Geometry: final body of the model. Coordinates: model frame, mm. Round coordinates to 2 decimals unless told otherwise and drop trailing zeros. Loops run counter-clockwise (first coordinate to the right, second up) from the corner with the lowest first, then second, coordinate; pieces in that order, holes last. Notation, with made-up numbers: (-25, 54.5) - (21, 54.5) arc R9 cw to (21, 70.5) - close; hole circle Ø5 at (32.25, 28). An arc over 180 degrees is marked (long way). Answer as a JSON object with one key per item and string values. Group by question number.
Item 1: Section A-A (z = 70.5). Return the cut outline in (x, y) (1 decimal).
Item 2: First-contact query: pin 1 (3 mm diameter, centred on y = -2, z = 101, fed in from +X); pin 2 (2 mm diameter, centred on x = 3.5, z = -84, fed in from +Y). Flat tips, straight axial feed; report the tip coordinate or a pass-through.
Item 3: Line query: line 1 (X direction, y = 0.25, z = 40.5); line 2 (Y direction, x = 0.75, z = 114); line 3 (X direction, y = -2.75, z = 89). Output: solid intervals per line, ascending.
```python
from build123d import *

# Parameters (mm, degrees)
SKETCH3_R                = 4.7625
BOSS_EXTRUDE2_DEPTH      = 152.4
BOSS_EXTRUDE2_DEPTH_BACK = 152.4
CUT_EXTRUDE5_DEPTH       = 153.4
CUT_EXTRUDE5_DEPTH_BACK  = 153.4
CHAMFER1_SIZE            = 0.47625


with BuildPart() as part:
    # Sketch3 → Boss-Extrude2 (new body, two sides)
    with BuildSketch(Plane.XY) as boss_extrude2_sk:
        Circle(SKETCH3_R)
    extrude(amount=BOSS_EXTRUDE2_DEPTH)
    extrude(boss_extrude2_sk.sketch, amount=-BOSS_EXTRUDE2_DEPTH_BACK)

    # Sketch10 → Cut-Extrude5 (cut, two sides)
    with BuildSketch(Plane.XY) as cut_extrude5_sk:
        with BuildLine():
            Line((-2.38125, 4.124445986), (2.38125, 4.124445986))
            ThreePointArc((2.38125, 4.124445986), (0, 4.7625), (-2.38125, 4.124445986))
        make_face()
    extrude(amount=CUT_EXTRUDE5_DEPTH, mode=Mode.SUBTRACT)
    extrude(cut_extrude5_sk.sketch, amount=-CUT_EXTRUDE5_DEPTH_BACK, mode=Mode.SUBTRACT)

    # Chamfer1
    chamfer1_edges = [part.edges().sort_by_distance(p)[0] for p in [
        (0, -4.7625, -152.4),
        (0, -4.7625, 152.4),
    ]]
    chamfer(chamfer1_edges, length=CHAMFER1_SIZE)


solid = part.part
```
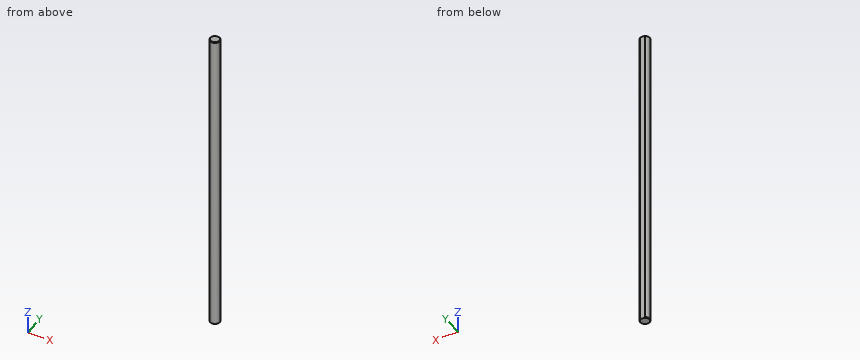
Values:
{
 "1": {"outline": "(-2.4, 4.1) arc R4.8 ccw (long way) to (2.4, 4.1) - close"},
 "2": {"pin 1": "stops at x = 4.74", "pin 2": "stops at y = 4.05"},
 "3": {"line 1": "x = -4.76 to 4.76", "line 2": "y = -4.7 to 4.12", "line 3": "x = -3.89 to 3.89"}
}
